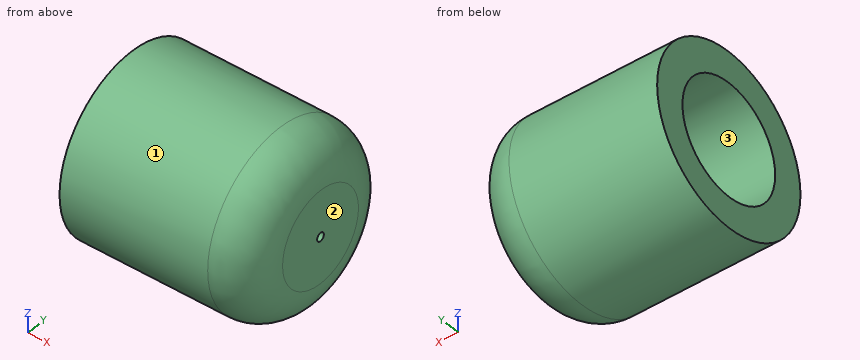
from build123d import *


with BuildPart() as f3:
    # F1 (on face) → F3 (revolve)
    with BuildSketch(Plane.XY):
        with BuildLine():
            Line((5, -2.75), (0, -2.75))
            Line((0, -2.75), (0, -4.25))
            Line((0, -4.25), (7.2, -4.25))
            ThreePointArc((7.2, -4.25), (8.614214, -3.664214), (9.2, -2.25))
            Line((9.2, -2.25), (9.2, -0.2))
            Line((9.2, -0.2), (8.2, -0.2))
            Line((8.2, -0.2), (8.2, -1.467218))
            ThreePointArc((8.2, -1.467218), (7.949678, -2.12902), (7.324035, -2.459496))
            Line((7.324035, -2.459496), (5, -2.75))
        make_face()
    revolve(axis=Axis((5.405035, 0, 0), (1, 0, 0)))


solid = f3.part
Build history of the part. All positions in model axes, mm. Face numbers are marked on the shaded views. Coordinates: 2 decimals unless noted, no trailing zeros. Order: outer loops, then holes, each group sorted by start corner. A loop starts at its lowest first (then second) coordinate and runs counter-clockwise, first axis right, second up. Notation, with made-up numbers: (6.25, 20) - (39.25, 20) arc R16 ccw to (39.25, 43) - close; hole circle Ø11 at (18, -20). An arc over 180 degrees is marked (long way). Write item = value, one per line. Start each with the question number.
1) Saw through at A-A on y = 0. Write the cut outline in (x, z).
2) Saw through at D-D on x = 6. Write the cut outline in (y, z) (3 decimals).
3) Wall check: line 1 along Y through (x, z) = (1.2, 0); line 2 along X through (y, z) = (-0.25, 1.25). Give the ranges that are in metal, low to high. Write a range as from..to.
4) Flat gauge pins, fed straight in: pin 1 Ø1.5 at (y, z) = (0, 0) entering from -X; pin 2 Ø1.5 at (x, z) = (6, -1.5) entering from +Y; pin 3 Ø1.5 at (x, z) = (7.5, -2.5) entering from -Y. Where does each tip first touch, or does it go through?
5) Saw through at C-C on x = 2. Write the cut outline in (y, z), then the cut area to 3 significant figures.
6) Two-plate mould, pull along Z, no slides. Class the marked faces 1, 2 and 3: pulls with the +Z half, pulls with the -Z half, needs draft (parallel to the pull), parting line crosses it, or undercut.
From the geometry:
q1.outline = (0, -4.25) - (7.2, -4.25) arc R2 ccw to (9.2, -2.25) - (9.2, -0.2) - (8.2, -0.2) - (8.2, -1.47) arc R1 cw to (7.32, -2.46) - (5, -2.75) - (0, -2.75) - close; (0, 2.75) - (5, 2.75) - (7.32, 2.46) arc R1 cw to (8.2, 1.47) - (8.2, 0.2) - (9.2, 0.2) - (9.2, 2.25) arc R2 ccw to (7.2, 4.25) - (0, 4.25) - close
q2.outline = circle Ø8.5 at (0, 0); hole circle Ø5.25 at (0, 0)
q3.line_1 = -4.25..-2.75, 2.75..4.25
q3.line_2 = 8.2..9.2
q4.pin_1 = 8.2
q4.pin_2 = 4.18
q4.pin_3 = -3.86
q5.outline = circle Ø8.5 at (0, 0); hole circle Ø5.5 at (0, 0)
q5.area = 33.0 mm^2
q6.face_1 = parting line crosses it
q6.face_2 = needs draft
q6.face_3 = undercut
